```python
from build123d import *

# Parameters (mm, degrees)
SKETCH1_R           = 5
BOSS_EXTRUDE1_DEPTH = 29
SKETCH2_R           = 4.8
BOSS_EXTRUDE2_DEPTH = 7.35
SKETCH3_R           = 4.305
BOSS_EXTRUDE3_DEPTH = 97
SKETCH4_R           = 2.75
BOSS_EXTRUDE4_DEPTH = 70
FILLET1_R           = 55
FILLET2_R           = 2.5


with BuildPart() as part:
    # Sketch1 → Boss-Extrude1 (new body)
    with BuildSketch(Plane(origin=(0, 0, 0), x_dir=(1, 0, 0), z_dir=(0, 1, 0))):
        with Locations(Location((0, 0, 0), (0, 0, 90))):
            Circle(SKETCH1_R)
    extrude(amount=BOSS_EXTRUDE1_DEPTH)

    # Sketch2 → Boss-Extrude2 (add)
    with BuildSketch(Plane.XY):
        with Locations(Location((0, 24.2, 0), (0, 0, 90))):
            Circle(SKETCH2_R)
    extrude(amount=BOSS_EXTRUDE2_DEPTH)

    # Sketch3 → Boss-Extrude3 (add)
    with BuildSketch(Plane.XY.offset(7.35)):
        with Locations(Location((0, 24.2, 0), (0, 0, 180))):
            Circle(SKETCH3_R)
    extrude(amount=BOSS_EXTRUDE3_DEPTH)

    # Sketch4 → Boss-Extrude4 (add)
    with BuildSketch(Plane.XY.offset(104.35)):
        with Locations((0, 24.2)):
            Circle(SKETCH4_R)
    extrude(amount=BOSS_EXTRUDE4_DEPTH)

    # Fillet1
    # the kernel refuses this fillet: 55 mm, written as the material it adds along each edge
    with BuildSketch(Plane(origin=(0, 24.2, 104.35), x_dir=(1, 0, 0), z_dir=(0, -1, 0))) as fillet1_piece_1:
        with BuildLine():
            CenterArc((57.75, 12.985837478), FILLET1_R, 180, 13.656834666)
            Line((2.75, 12.985837478), (1.65, 12.985837478))
            Line((1.65, 12.985837478), (1.65, 0))
            Line((1.65, 0), (2.75, -1.1))
            ThreePointArc((2.75, -1.1), (3.5275, -1.1), (3.2361, -0.25971675))
            Line((3.2361, -0.25971675), (4.305, 0))
        make_face()
    revolve(axis=Axis((0, 24.2, 104.35), (0, 0, 1)))

    # Fillet2
    # the kernel refuses this fillet: 2.5 mm, written as the material it adds along each edge
    with BuildSketch(Plane(origin=(0, 24.2, 7.35), x_dir=(-1, 0, 0), z_dir=(0, 1, 0))) as fillet2_piece_1:
        with BuildLine():
            CenterArc((6.805, 1.493310082), FILLET2_R, 180, 36.678485047)
            Line((4.8, 0), (4.7599, -0.029866202))
            ThreePointArc((4.7599, -0.029866202), (4.5525, -0.05), (4.305, -0.05))
            Line((4.305, -0.05), (4.255, 0))
            Line((4.255, 0), (4.255, 1.493310082))
            Line((4.255, 1.493310082), (4.305, 1.493310082))
        make_face()
    revolve(axis=Axis((0, 24.2, 7.35), (0, 0, 1)))


solid = part.part
```
Verification items for the finished model (mm, model axes). A direction names the side the tool comes from. Round coordinates to 2 decimals unless told otherwise and drop trailing zeros. Write each loop counter-clockwise with the first axis right and the second up, starting at its lowest first coordinate (ties: lowest second). Pieces come first, ordered by that corner, then holes. Notation, with made-up numbers: (0, 32.25) - (23, 32.25) arc R22 ccw to (23, 50.25) - close; hole circle Ø6 at (81.25, -18). An arc over 180 degrees is marked (long way). Answer as a JSON object with one key per item and string values. Group by question number.
Q1. Section check A-A, the plane y = 24.2. Enter the section's corners in (x, z) (3 decimals), plus the area to 3 significant figures.
Q2. Go/stop test with flat-tipped pins: pin 1 Ø1 at (x, y) = (3, 9) entering from +Z; pin 2 Ø4 at (x, z) = (-4, 117.5) entering from +Y; pin 3 Ø4 at (x, z) = (2.5, 57.5) entering from -Y. Record where each tip stops, or that it passes through.
Q3. Section check B-B, the plane y = 8. Enter the section's corners in (x, z).
Q4. Tool access check on faces 1 (the flat face through (0, 29, 0)), 2 (the cylindrical face through (-0.358, 26.927, 145.444)). Record the directions out of +Z, -Z, +X, -X, +Y, -Y that give a thin tool (end or side, any length) a straight path to the whole face; none if there is none.
Q5. Thickness scan on line 1 (Z direction, x = 2.5, y = 19); line 2 (X direction, y = 24.75, z = 100); line 3 (Z direction, x = -0.25, y = 13). Record the ranges inside material, lowest first.
Found:
{
 "1": {"outline": "(-4.8, 1.4) arc R5 ccw (long way) to (4.8, 1.4) - (4.8, 7.35) arc R2.5 cw to (4.305, 8.843) - (4.305, 104.35) arc R55 cw to (2.75, 117.336) - (2.75, 174.35) - (-2.75, 174.35) - (-2.75, 117.336) arc R55 cw to (-4.305, 104.35) - (-4.305, 8.843) arc R2.5 cw to (-4.8, 7.35) - close", "area": "1,340 mm^2"},
 "2": {"pin 1": "stops at z = 4.33", "pin 2": "stops at y = 26.09", "pin 3": "stops at y = 19.92"},
 "3": {"outline": "circle Ø10 at (0, 0)"},
 "4": {"face 1": "+Z, -Z, +X, -X, +Y", "face 2": "+Z"},
 "5": {"line 1": "z = -4.33 to 4.33", "line 2": "x = -4.27 to 4.27", "line 3": "z = -4.99 to 4.99"}
}
